```python
from build123d import *

# Parameters (mm, degrees)
F0_R      = 2.125
F1_DEPTH  = 5
F3_DEPTH  = 20
F4_R      = 2.125
F5_DEPTH  = 5
F7_DEPTH  = 5
F8_R      = 1.5
F9_R      = 2.125
F10_DEPTH = 25


with BuildPart() as f1:
    # F0 (on Top) → F1 (new body)
    with BuildSketch(Plane.XY):
        Polygon((0, 25), (0, 50), (-25, 50), (-25, 0), (25, 0), (25, 25), align=None)
        with Locations((-12.5, 12.5)):
            Circle(F0_R, mode=Mode.SUBTRACT)
        with Locations((15, 12.5)):
            Circle(F0_R, mode=Mode.SUBTRACT)
        with Locations((-12.5, 40)):
            Circle(F0_R, mode=Mode.SUBTRACT)
    extrude(amount=F1_DEPTH)

    # F2 (on face) → F3 (join)
    with BuildSketch(Plane.XY.offset(5)):
        Polygon((25, 5), (-20, 5), (-20, 50), (-25, 50), (-25, 0), (-20, 0), (25, 0), align=None)
    extrude(amount=F3_DEPTH)

    # F4 (on face) → F5 (cut)
    with BuildSketch(Plane.XZ):
        with Locations((10, 12.5)):
            Circle(F4_R)
    extrude(amount=-F5_DEPTH, mode=Mode.SUBTRACT)

    # F6 (on Top) → F7 (join)
    with BuildSketch(Plane.XY):
        Polygon((25, 25), (0, 50), (0, 25), align=None)
    extrude(amount=F7_DEPTH)

    # F8
    f8_edges = [f1.edges().sort_by_distance(p)[0] for p in [
        (-25, 0, 12.5),
    ]]
    fillet(f8_edges, radius=F8_R)

    # F9 (on face) → F10 (cut)
    with BuildSketch(Plane(origin=(-25, 0, 0), x_dir=(0, -1, 0), z_dir=(-1, 0, 0))):
        with Locations((-35, 12.5)):
            Circle(F9_R)
    extrude(amount=-F10_DEPTH, mode=Mode.SUBTRACT)


solid = f1.part
```
Geometry: final body of the model. Coordinates: model frame, mm. A direction names the side the tool comes from. Round coordinates to 2 decimals unless told otherwise and drop trailing zeros. Order: outer loops, then holes, each group sorted by start corner. A loop starts at its lowest first (then second) coordinate and runs counter-clockwise, first axis right, second up. Notation, with made-up numbers: (71, 78.5) - (106, 78.5) arc R21 ccw to (106, 109.5) - close; hole circle Ø11 at (63, 62.5). An arc over 180 degrees is marked (long way). Write item = value, one per line. Start each with the question number.
Q1. Pull-direction query (Y, two-part tool) for faces 3 (the flat face through (25, 7, 4)), 4 (the cylindrical face through (-22.535, 32.973, 13.138)), 5 (the cylindrical face through (12.877, 12.593, 2.465)), 6 (the flat face through (13, 37, 2)); classes: +Y half, -Y half, draft (parallel to the pull), parting line (faces both ways), or undercut.
Q2. Ray query, line 1 (Z direction, x = 10, y = 3) (3 decimals); line 2 (X direction, y = 11.5, z = 8); line 3 (Z direction, x = -5, y = 30.5). Return the intervals inside material, ascending. Write a range as from..to.
Q3. Cut plane A-A on y = 35. Return the cut outline in (x, z) (3 decimals), and give its area (3 significant figures).
Q4. Cut plane C-C on z = 12.5. Return the cut outline in (x, y) (3 decimals), and give its area (3 significant figures).
Q5. Cut plane B-B on x = 15. Return the cut outline in (y, z) (3 decimals).
Q6. Pin query (flat end, axial travel): pin 1 (1.5 mm diameter, centred on x = -9, z = 14.5, fed in from +Y); pin 2 (5 mm diameter, centred on y = 26.5, z = 10.5, fed in from +X); pin 3 (12 mm diameter, centred on y = 40, z = 7.5, fed in from +X). Return the tip coordinate at first contact, or that it passes through.
Q7. Cut plane D-D on y = 12.5. Return the cut outline in (x, z) (3 decimals).
Q8. Access query for faces 1 (the flat face through (0, 0, 12)), 2 (the flat face through (3, 5, 15)). Directions: +Z, -Z, +X, -X, +Y, -Y. A direction counts if a zero-diameter tool reaches every point of the face in a straight line with its end or side. Return the directions, or none.
Outcome:
q1.face_3 = draft
q1.face_4 = undercut
q1.face_5 = undercut
q1.face_6 = +Y half
q2.line_1 = 0..10.375, 14.625..25
q2.line_2 = -25..-20
q2.line_3 = 0..5
q3.outline = (-25, 0) - (15, 0) - (15, 5) - (-20, 5) - (-20, 10.375) - (-25, 10.375) - close; (-25, 14.625) - (-20, 14.625) - (-20, 25) - (-25, 25) - close
q3.area = 279 mm^2
q4.outline = (-25, 1.5) arc R1.5 ccw to (-23.5, 0) - (7.875, 0) - (7.875, 5) - (-20, 5) - (-20, 32.875) - (-25, 32.875) - close; (-25, 37.125) - (-20, 37.125) - (-20, 50) - (-25, 50) - close; (12.125, 0) - (25, 0) - (25, 5) - (12.125, 5) - close
q4.area = 432 mm^2
q5.outline = (0, 0) - (10.375, 0) - (10.375, 5) - (5, 5) - (5, 25) - (0, 25) - close; (14.625, 0) - (35, 0) - (35, 5) - (14.625, 5) - close
q6.pin_1 = 5
q6.pin_2 = -20
q6.pin_3 = 15.45
q7.outline = (-25, 0) - (-14.625, 0) - (-14.625, 5) - (-20, 5) - (-20, 25) - (-25, 25) - close; (-10.375, 0) - (12.875, 0) - (12.875, 5) - (-10.375, 5) - close; (17.125, 0) - (25, 0) - (25, 5) - (17.125, 5) - close
q8.face_1 = +Z, -Z, +X, -X, -Y
q8.face_2 = +Z, +X, +Y
